Print and shaded views of the part. All mm, measured from the part's lowest x, y and z. A direction names the side the tool comes from. Round coordinates to 2 decimals unless told otherwise and drop trailing zeros. Loops run counter-clockwise (first coordinate to the right, second up) from the corner with the lowest first, then second, coordinate; pieces in that order, holes last. Notation, with made-up numbers: (65, -30) -> (121, -30) arc R37 ccw to (121, 6) -> close; hole circle Ø10 at (-32, 82). An arc over 180 degrees is marked (long way). Answer as CSV lines item,"result".
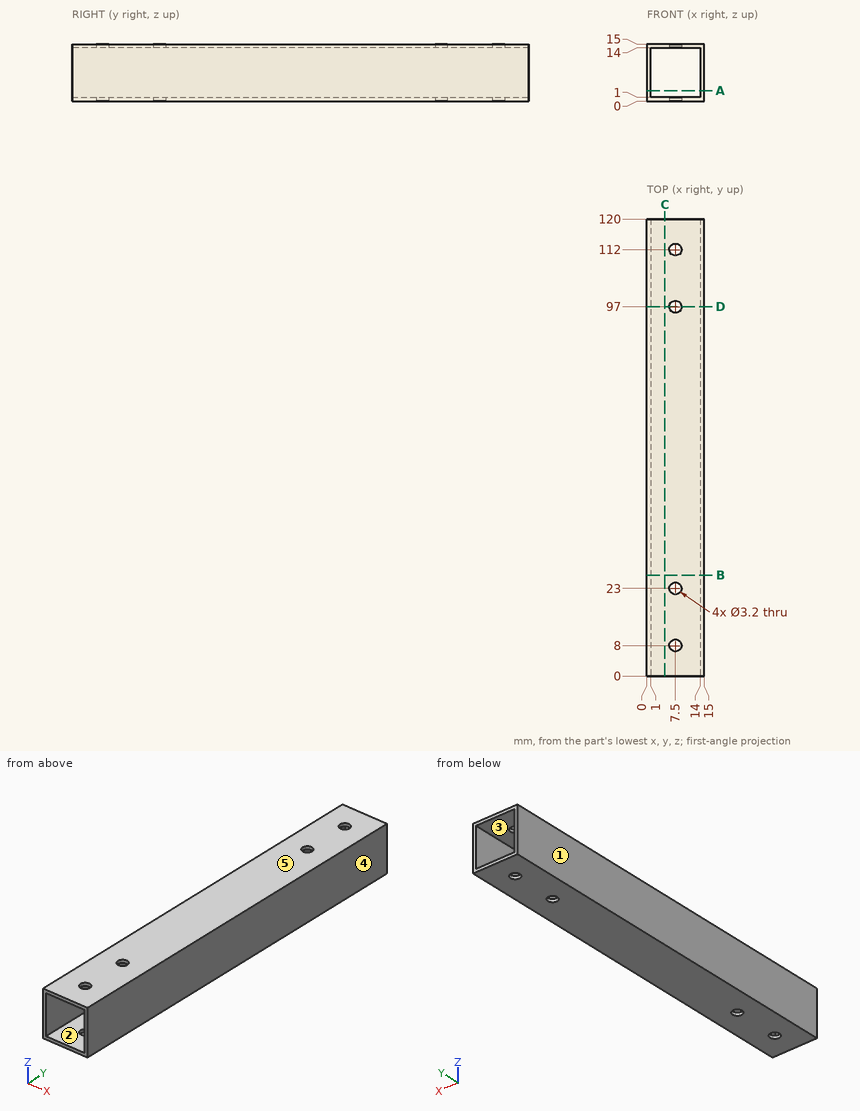
Q1. Two-plate mould, pull along X, no slides. Class the marked faces 3, 4 and 5: pulls with the +X half, pulls with the -X half, needs draft (parallel to the pull), parting line crosses it, or undercut.
Geometry results:
face 3,"undercut"
face 4,"pulls with the +X half"
face 5,"needs draft"
Q2. Saw through at A-A, the plane z = 2.75. Write the cut outline in (x, y), then the cut area to 3 significant figures.
Geometry results:
outline,"(0, 0) -> (1, 0) -> (1, 120) -> (0, 120) -> close; (14, 0) -> (15, 0) -> (15, 120) -> (14, 120) -> close"
area,"240 mm2"
Q3. Drill centre lines: line 1 along Y through (x, z) = (7.5, 0.85); line 2 along X through (y, z) = (68, 5.5). Where is each one in solid material? Low to high.
Geometry results:
line 1,"0 to 6.4, 9.6 to 21.4, 24.6 to 95.4, 98.6 to 110.4, 113.6 to 120"
line 2,"0 to 1, 14 to 15"
Q4. Saw through at D-D, the plane y = 97. Write the cut outline in (x, z).
Geometry results:
outline,"(0, 0) -> (5.9, 0) -> (5.9, 1) -> (1, 1) -> (1, 14) -> (5.9, 14) -> (5.9, 15) -> (0, 15) -> close; (9.1, 0) -> (15, 0) -> (15, 15) -> (9.1, 15) -> (9.1, 14) -> (14, 14) -> (14, 1) -> (9.1, 1) -> close"
Q5. Saw through at C-C, the plane x = 4.75. Write the cut outline in (y, z).
Geometry results:
outline,"(0, 0) -> (120, 0) -> (120, 1) -> (0, 1) -> close; (0, 14) -> (120, 14) -> (120, 15) -> (0, 15) -> close"
Q6. Which spindle directions (+Z, -Z, +X, -X, +Y, -Y) get a long thin tool onto all of the face, cutting with end or side? Do the marked faces 1 and 2. Say none if no direction does.
Geometry results:
face 1,"+Z, -Z, -X, +Y, -Y"
face 2,"+Y, -Y"
Q7. Saw through at B-B, the plane y = 26.5. Write the cut outline in (x, z), then the cut area to 3 significant figures.
Geometry results:
outline,"(0, 0) -> (15, 0) -> (15, 15) -> (0, 15) -> close; hole (1, 1) -> (14, 1) -> (14, 14) -> (1, 14) -> close"
area,"56.0 mm2"
